Could you check a few things on this model? Use its own coordinates, in mm. Face numbers are marked on the shaded views. A direction names the side the tool comes from. Round coordinates to 2 decimals unless told otherwise and drop trailing zeros. Loops run counter-clockwise (first coordinate to the right, second up) from the corner with the lowest first, then second, coordinate; pieces in that order, holes last.
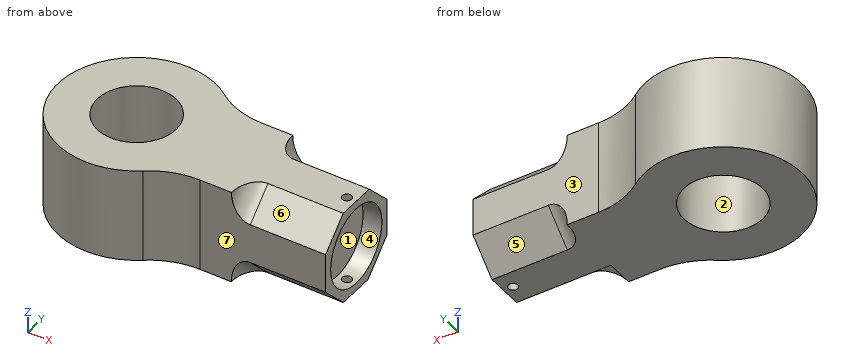
from build123d import *

# Parameters (mm, degrees)
SKETCH1_R              = 250
BOSS_EXTRUDE1_DEPTH    = 600
CUT_EXTRUDE6_DEPTH     = 600
CUT_EXTRUDE8_START     = -1
CUT_EXTRUDE8_OUTLINE_W = 600
CUT_EXTRUDE8_OUTLINE_H = 174.000412652
CUT_EXTRUDE8_DEPTH     = 1
FILLET2_R              = 120
SKETCH8_R              = 250
CUT_EXTRUDE10_DEPTH    = 120
SKETCH9_R              = 30
CUT_EXTRUDE11_DEPTH    = 1604.121954188


# Read off the part's stored shape, not the designer's step: Cut-Extrude8
with BuildPart() as part:
    # Sketch1 → Boss-Extrude1 (new body)
    with BuildSketch(Plane.XY):
        with BuildLine():
            Line((600, 300), (1400, 300))
            Line((1400, 300), (1400, -300))
            Line((1400, -300), (600, -300))
            ThreePointArc((600, -300), (441.886116992, -325.658350975), (300, -400))
            ThreePointArc((300, -400), (-500, 0), (300, 400))
            ThreePointArc((300, 400), (441.886116992, 325.658350975), (600, 300))
        make_face()
        Circle(SKETCH1_R, mode=Mode.SUBTRACT)
    extrude(amount=BOSS_EXTRUDE1_DEPTH)

    # Sketch2 → Cut-Extrude6 (cut)
    with BuildSketch(Plane(origin=(1400, 0, 0), x_dir=(0, 0, -1), z_dir=(1, 0, 0))):
        Polygon((-180.6, 300), (0, 114), (0, 300), align=None)
        Polygon((-600, -300), (-432.420494682, -300), (-600, -127.409811799), align=None)
        Polygon((-0.445053521, -300), (-0.445053521, -125.999587348), (-179.648136318, -300), align=None)
        Polygon((-606.599587348, 119.845053521), (-606.599587348, 300.445053521), (-420.599587348, 300.445053521), align=None)
    extrude(amount=-CUT_EXTRUDE6_DEPTH, mode=Mode.SUBTRACT)

    # Cut-Extrude8 outline → Cut-Extrude8 (cut)
    with BuildSketch(Plane(origin=(0, 0, 0), x_dir=(-1, 0, 0), z_dir=(0, 0, -1)).offset(CUT_EXTRUDE8_START)):
        with Locations((-1100, -212.999793674)):
            Rectangle(CUT_EXTRUDE8_OUTLINE_W, CUT_EXTRUDE8_OUTLINE_H)
    extrude(amount=CUT_EXTRUDE8_DEPTH, mode=Mode.SUBTRACT)

    # Fillet2
    fillet2_edges = [part.edges().sort_by_distance(p)[0] for p in [
        (800, 213.126519973, 510.528974059),
        (800, -213.269211239, 90.324068159),
        (800, -213.7049059, 516.210247341),
        (800, 207, 90.3),
    ]]
    fillet(fillet2_edges, radius=FILLET2_R)

    # Sketch8 → Cut-Extrude10 (cut)
    with BuildSketch(Plane(origin=(1400, 0, 0), x_dir=(0, 0, -1), z_dir=(1, 0, 0))):
        with Locations((-300, 0)):
            Circle(SKETCH8_R)
    extrude(amount=-CUT_EXTRUDE10_DEPTH, mode=Mode.SUBTRACT)

    # Sketch9 → Cut-Extrude11 (cut, through all)
    with BuildSketch(Plane(origin=(0, 0, 0), x_dir=(-1, 0, 0), z_dir=(0, 0, -1))):
        with Locations((-1340, 0)):
            Circle(SKETCH9_R)
    extrude(amount=-CUT_EXTRUDE11_DEPTH, mode=Mode.SUBTRACT)


solid = part.part
Item 1: If we section it at A-A, the plane x = 0: Please give me the cut outline in (y, z).
Results list:
outline: (-500, 0) - (-250, 0) - (-250, 600) - (-500, 600) - close; (250, 0) - (500, 0) - (500, 600) - (250, 600) - close
Item 2: We'd pull the mould along X, two halves only. Please class the marked faces 1, 2 and 3: released by +X, released by -X, zero draft, split by the parting line, or undercut.
Results list:
face 1: released by +X
face 2: undercut
face 3: zero draft
Item 3: Will these pins go through, and if not, where does the flat tip stop? pin 1 (2 mm diameter, centred on x = 289.5, z = 469.5, fed in from +Y); pin 2 (1 mm diameter, centred on x = 33.5, z = 137.5, fed in from -Y); pin 3 (6 mm diameter, centred on y = 267.5, z = 460, fed in from -X).
Results list:
pin 1: stops at y = 408.37
pin 2: stops at y = -498.91
pin 3: stops at x = -424.31
Item 4: If we section it at D-D, the plane x = 1128: Please give me the cut outline in (y, z).
Results list:
outline: (-300, 179.65) - (-126.54, 1) - (-126, 1) - (-126, 0) - (114, 0) - (300, 180.6) - (300, 421.06) - (126.25, 600) - (-127.41, 600) - (-300, 432.42) - close
Item 5: If I drill on line 1 along Y through (x, z) = (-7.5, 33); line 2 along Y through (x, z) = (1365, 300); line 3 along X through (y, z) = (56, 165), over which ranges is the centre line in solid material (lowest first)?
Results list:
line 1: y = -499.94 to -249.89, 249.89 to 499.94
line 2: y = -300 to -250, 250 to 300
line 3: x = -496.85 to -243.65, 243.65 to 1280
Item 6: For the marked faces 4, 5, 6 and 7, which set-ups out of +Z, -Z, +X, -X, +Y, -Y let a thin tool reach every point of the face, with its end or its side?
Results list:
face 4: +X
face 5: -Z, +X, +Y
face 6: +Z, +X, -Y
face 7: +Z, -Z, +X, -Y
Item 7: If we section it at B-B, the plane y = 0: Please give me the cut outline in (x, z), then the cut area to 3 significant figures.
Results list:
outline: (-500, 0) - (-250, 0) - (-250, 600) - (-500, 600) - close; (250, 0) - (1310, 0) - (1310, 50) - (1280, 50) - (1280, 550) - (1310, 550) - (1310, 600) - (250, 600) - close; (1370, 0) - (1400, 0) - (1400, 50) - (1370, 50) - close; (1370, 550) - (1400, 550) - (1400, 600) - (1370, 600) - close
area: 774,000 mm2
Item 8: If we section it at C-C, the plane z = 300: Please give me the cut outline in (x, y), then the cut area to 3 significant figures.
Results list:
outline: (300, -400) arc R500 cw to (600, -300) - (1400, -300) - (1400, -250) - (1280, -250) - (1280, 250) - (1400, 250) - (1400, 300) - (600, 300) arc R500 cw to (300, 400) arc R500 ccw (long way) to start; hole circle Ø500 at (0, 0)
area: 1,100,000 mm2
